```python
from build123d import *

# Parameters (mm, degrees)
EXTRUDE_1_DEPTH     = 4
SKETCH_2_R          = 2.5
CUT_EXTRUDE_1_DEPTH = 5


with BuildPart() as part:
    # Эскиз1 → Бобышка-Вытянуть1 (new body)
    with BuildSketch(Plane.XY):
        Polygon((87.193826731, -36.850553491), (87.193826731, -86.850553491), (187.193824318, -86.828585686), (187.193824318, -6.828585686), (110.85, 53.001797886), (6, 53.001797886), (-4, 53.001797886), (-4, 23.001797886), (2, 23.001797886), (2, 43.001797886), (5.711449025, 43.001797886), (5.711449025, -16.998202114), (64.208325653, -16.998202114), align=None)
    extrude(amount=EXTRUDE_1_DEPTH)

    # Эскиз2 → Вырез-Вытянуть1 (cut, through all)
    with BuildSketch(Plane.XY.offset(4)):
        with Locations((112.19490079, -81.850553491)):
            Circle(SKETCH_2_R)
        with Locations((162.19490079, -81.850553491)):
            Circle(SKETCH_2_R)
    extrude(amount=-CUT_EXTRUDE_1_DEPTH, mode=Mode.SUBTRACT)


solid = part.part
```
For this review, take the finished solid that the model builds, in its own axes (mm). A direction names the side the tool comes from. Give positions to 0.01 mm unless a question says otherwise; leave off trailing zeros. Order: outer loops, then holes, each group sorted by start corner. A loop starts at its lowest first (then second) coordinate and runs counter-clockwise, first axis right, second up.
1) Take a section at D-D (y = -39.5). Give the boundary of the cut face in (x, z).
2) For faces 4 (the face through (187.194, -47, 2)), 5 (the face through (35, -16.998, 2)), 6 (the face through (4, 43.002, 2)), list the 3-axis set-ups (+Z, -Z, +X, -X, +Y, -Y) from which the entire face can be reached by the end or side of a thin tool; tool diameter is ignored.
3) Insertion check: pin 1 (1.1 mm diameter, centred on x = 4, z = 1.5, fed in from -Y); pin 2 (1.2 mm diameter, centred on y = 35, z = 3, fed in from +X); pin 3 (3 mm diameter, centred on x = 162.19, y = -81.85, fed in from +Z); pin 4 (2 mm diameter, centred on y = -61.5, z = 1, fed in from -X). Each pin has a flat end and moves straight along its axis. Give the tip position at first contact, or say it passes through.
4) Take a section at B-B (z = 2.6). Give the boundary of the cut face in (x, y).
5) The part is to be moulded in two halves that separate along Y. For faces 1 (the face through (161.7, -84.3, 2)), 2 (the face through (112, -16, 0)), 3 (the face through (-1, 23.002, 2)), say which applies: released by +Y, released by -Y, zero draft, split by the parting line, or undercut.
6) Wall thickness on line 1 (Y direction, x = 57, z = 1.85); line 2 (X direction, y = 24, z = 1.15); line 3 (X direction, y = -66, z = 0.7): over which ranges is each line inside the solid? List them lowest first.
7) Take a section at A-A (y = 27.5). Give the boundary of the cut face in (x, z).
8) Take a section at C-C (x = 32.5). Give the boundary of the cut face in (y, z).
Derived:
1. outline: (87.19, 0) - (187.19, 0) - (187.19, 4) - (87.19, 4) - close
2. face 4: +Z, -Z, +X, +Y, -Y
2. face 5: +Z, -Z, -X, -Y
2. face 6: +Z, -Z, -Y
3. pin 1: stops at y = 43
3. pin 2: stops at x = 134.59
3. pin 3: passes through
3. pin 4: stops at x = 87.19
4. outline: (-4, 23) - (2, 23) - (2, 43) - (5.71, 43) - (5.71, -17) - (64.21, -17) - (87.19, -36.85) - (87.19, -86.85) - (187.19, -86.83) - (187.19, -6.83) - (110.85, 53) - (-4, 53) - close; hole circle Ø5 at (112.19, -81.85); hole circle Ø5 at (162.19, -81.85)
5. face 1: undercut
5. face 2: zero draft
5. face 3: released by -Y
6. line 1: y = -17 to 53
6. line 2: x = -4 to 2, 5.71 to 147.86
6. line 3: x = 87.19 to 187.19
7. outline: (-4, 0) - (2, 0) - (2, 4) - (-4, 4) - close; (5.71, 0) - (143.39, 0) - (143.39, 4) - (5.71, 4) - close
8. outline: (-17, 0) - (53, 0) - (53, 4) - (-17, 4) - close
